Work out the finished part from the listing and answer in its coordinate system (mm). A direction names the side the tool comes from. Coordinates: 2 decimals unless noted, no trailing zeros. Loops run counter-clockwise (first coordinate to the right, second up) from the corner with the lowest first, then second, coordinate; pieces in that order, holes last. Notation, with made-up numbers: (-31.5, 56.25) -> (-22.5, 56.25) arc R21 cw to (-22.5, 78.25) -> close; hole circle Ø2 at (-37, 77.25). An arc over 180 degrees is marked (long way). Use a Markdown table: item, result. Add a question column.
```python
from build123d import *

# Parameters (mm, degrees)
F0_W     = 60
F0_H     = 260
F0_R     = 7.5
F1_DEPTH = 40
F0_W_2   = 200
F2_DEPTH = 94
F4_DEPTH = 200
F5_R     = 75
F6_DEPTH = 324.75
F7_R     = 5


with BuildPart() as f1:
    # F0 (on Top) → F1 (new body)
    with BuildSketch(Plane.XY):
        with Locations((130, 0)):
            Rectangle(F0_W, F0_H)
        with Locations((130, -80)):
            Circle(F0_R, mode=Mode.SUBTRACT)
        with Locations((130, 60)):
            Circle(F0_R, mode=Mode.SUBTRACT)
    extrude(amount=F1_DEPTH)



with BuildPart() as f1b:
    # F0 (on Top) → F1, piece 2 (new body)
    with BuildSketch(Plane.XY):
        with Locations((-130, 0)):
            Rectangle(F0_W, F0_H)
        with Locations((-130, -80)):
            Circle(F0_R, mode=Mode.SUBTRACT)
        with Locations((-130, 60)):
            Circle(F0_R, mode=Mode.SUBTRACT)
    extrude(amount=F1_DEPTH)


with BuildPart() as f1_1:
    add(f1.part)

    add(f1b.part)  # F2 merges F1b
    # F0 (on Top) → F2 (join)
    with BuildSketch(Plane.XY):
        Rectangle(F0_W_2, F0_H)
    extrude(amount=F2_DEPTH)

    # F3 (on face) → F4 (join)
    with BuildSketch(Plane.YZ.offset(100)):
        Polygon((20, 244), (-130, 94), (130, 94), (130, 164), (70, 244), align=None)
    extrude(amount=-F4_DEPTH)

    # F5 (on face) → F6 (cut)
    with BuildSketch(Plane(origin=(0, -112, 112), x_dir=(1, 0, 0), z_dir=(0, -0.7071067812, 0.7071067812))):
        with Locations((0, 94.4373130938)):
            Circle(F5_R)
    extrude(amount=-F6_DEPTH, mode=Mode.SUBTRACT)

    # F7
    f7_edges = [f1_1.edges().sort_by_distance(p)[0] for p in [
        (-160, -130, 20),
        (160, -130, 20),
        (160, 130, 20),
        (-160, 130, 20),
    ]]
    fillet(f7_edges, radius=F7_R)


solid = f1_1.part
```
Item 1: Section B-B (x = -9.5) is taken. Determine the outline of the cut face in (y, z), then the cut area to 3 significant figures.
Item 2: Section C-C (y = -80) is taken. Count the separate pieces of the cut face and the enclosed holes in it, then the cut area to 3 significant figures.
Item 3: Given pin 1 (18 mm diameter, centred on x = -143, y = -39, fed in from +Z); pin 2 (1.5 mm diameter, centred on y = -24.5, z = 65.5, fed in from -X); pin 3 (1 mm diameter, centred on y = -23, z = 192.5, fed in from +X), each flat-ended and moving along its own axis, determine where each tip first touches the part or whether it passes through.
Item 4: Find the intervals of material crossed by probe 1 along Y at (x, z) = (130, 28); probe 2 along Y at (x, z) = (29, 116); probe 3 along X at (y, z) = (68.5, 180), in increasing order.
Item 5: For faces 5 (the face through (-100, 27, 121)), 6 (the face through (100, 27, 121)), 7 (the face through (-160, -2, 20)), determine the directions among +Z, -Z, +X, -X, +Y, -Y from which every point of the face is accessible in a straight line to the end or side of a thin tool.
Item 6: Section A-A (x = -130) is taken. Determine the outline of the cut face in (y, z).
Item 7: For a pull along Y with two mould halves and no side action, classify faces 1 (the face through (-130, 2, 40)), 2 (the face through (-2, -130, 36)), 3 (the face through (1.4, 100.42, 203.44)), 4 (the face through (-122.846, 62.253, 19.72)) as +Y half, -Y half, draft (parallel to the pull), parting line (faces both ways), or undercut.
Output:
| question | item | result |
|---|---|---|
| 1 | outline | (-130, 0) -> (28.34, 0) -> (-97.83, 126.17) -> (-130, 94) -> close; (7.38, 231.38) -> (130, 108.77) -> (130, 164) -> (70, 244) -> (20, 244) -> close |
| 1 | area | 18,100 mm2 |
| 2 | separate pieces | 3 |
| 2 | enclosed holes | 0 |
| 2 | area | 29,500 mm2 |
| 3 | pin 1 | stops at z = 40 |
| 3 | pin 2 | stops at x = -100 |
| 3 | pin 3 | stops at x = 100 |
| 4 | probe 1 | y = -130 to -87.5, -72.5 to 52.5, 67.5 to 130 |
| 4 | probe 2 | y = -108 to -80.26, 115.37 to 130 |
| 4 | probe 3 | x = -100 to 100 |
| 5 | face 5 | +Z, -X, +Y, -Y |
| 5 | face 6 | +Z, +X, +Y, -Y |
| 5 | face 7 | +Z, -Z, -X, +Y, -Y |
| 6 | outline | (-130, 0) -> (-87.5, 0) -> (-87.5, 40) -> (-130, 40) -> close; (-72.5, 0) -> (52.5, 0) -> (52.5, 40) -> (-72.5, 40) -> close; (67.5, 0) -> (130, 0) -> (130, 40) -> (67.5, 40) -> close |
| 7 | face 1 | draft |
| 7 | face 2 | -Y half |
| 7 | face 3 | +Y half |
| 7 | face 4 | undercut |
